Check sheet for the modelled part. Datum: model origin and axes. Units: mm. A direction names the side the tool comes from. Round coordinates to 2 decimals unless told otherwise and drop trailing zeros. Loops run counter-clockwise (first coordinate to the right, second up) from the corner with the lowest first, then second, coordinate; pieces in that order, holes last. Notation, with made-up numbers: (-29, 48) -> (-24, 48) arc R20 cw to (-24, 54) -> close; hole circle Ø6 at (77.5, 87.5). An arc over 180 degrees is marked (long way). Return JSON: item names as keys, results as strings.
from build123d import *

# Parameters (mm, degrees)
SKETCH_1_W                        = 13
SKETCH_1_H                        = 30
SM_BASE_FLANGE_1_DEPTH            = 1
SM_EDGE_FLANGE_1_STRIP_W          = 6
SM_EDGE_FLANGE_1_STRIP_H          = 1
SM_EDGE_FLANGE_1_STRIP_CUT_DEPTH  = 10
SM_EDGE_FLANGE_1_RELIEF_W         = 6.5
SM_EDGE_FLANGE_1_RELIEF_H         = 0.5
SM_EDGE_FLANGE_1_RELIEF_CUT_DEPTH = 1
SM_EDGE_FLANGE_1_DEPTH            = 10
SM_EDGE_FLANGE_1_PROFILE_R        = 1
SM_EDGE_FLANGE_1_PROFILE_R_2      = 0.75
SM_EDGE_FLANGE_1_FLAT_DEPTH       = 1
FILLET_1_R                        = 3
SKETCH_9_R                        = 1.6
CUT_EXTRUDE_1_DEPTH               = 18.615014781


# Sheet-metal steps are written as plain solids
with BuildPart() as part:
    # Sketch 1 → 基体-法兰1 (new body)
    with BuildSketch(Plane.XY):
        Rectangle(SKETCH_1_W, SKETCH_1_H)
    extrude(amount=-SM_BASE_FLANGE_1_DEPTH)

    # 边线-法兰1 strip (across the edge) → 边线-法兰1 strip cut (cut)
    with BuildSketch(Plane(origin=(-6.5, 5, -1), x_dir=(1, 0, 0), z_dir=(0, 1, 0))):
        with Locations((-1, -0.5)):
            Rectangle(SM_EDGE_FLANGE_1_STRIP_W, SM_EDGE_FLANGE_1_STRIP_H)
    sm_edge_flange_1_strip_cut = extrude(amount=SM_EDGE_FLANGE_1_STRIP_CUT_DEPTH, mode=Mode.SUBTRACT)

    # 边线-法兰1 relief (on the sheet) → 边线-法兰1 relief cut (cut)
    with BuildSketch(Plane(origin=(-4.5, 5, -1), x_dir=(1, 0, 0), z_dir=(0, 0, -1))):
        with Locations((-2.75, 0.25)):
            Rectangle(SM_EDGE_FLANGE_1_RELIEF_W, SM_EDGE_FLANGE_1_RELIEF_H)
    sm_edge_flange_1_relief_cut = extrude(amount=-SM_EDGE_FLANGE_1_RELIEF_CUT_DEPTH, mode=Mode.SUBTRACT)

    # 边线-法兰1 bend section (across the edge) → 边线-法兰1 (add)
    with BuildSketch(Plane(origin=(-6.5, 5, -1), x_dir=(1, 0, 0), z_dir=(0, 1, 0))):
        with BuildLine():
            Line((0, 1), (1, 1))
            ThreePointArc((1, 1), (1.292893219, 0.292893219), (2, 0))
            Line((2, 0), (2, -1))
            ThreePointArc((2, -1), (0.585786438, -0.414213562), (0, 1))
        make_face()
    sm_edge_flange_1 = extrude(amount=SM_EDGE_FLANGE_1_DEPTH)

    # 边线-法兰1 profile (on flange) → 边线-法兰1 flat (add)
    with BuildSketch(Plane(origin=(-6.5, 0, -1), x_dir=(0, -1, 0), z_dir=(1, 0, 0))):
        with BuildLine():
            Line((-15, 1), (-5, 1))
            Line((-5, 1), (-5, 3.360392195))
            ThreePointArc((-5, 3.360392195), (-5.453315717, 4.628370006), (-6.60776773, 5.321553546))
            Line((-6.60776773, 5.321553546), (-12.60776773, 6.521553546))
            ThreePointArc((-12.60776773, 6.521553546), (-14.267977811, 6.107076477), (-15, 4.560392195))
            Line((-15, 4.560392195), (-15, 1))
        make_face()
        with Locations((-13, 2.5)):
            Circle(SM_EDGE_FLANGE_1_PROFILE_R, mode=Mode.SUBTRACT)
        with Locations((-7, 3.360392195)):
            Circle(SM_EDGE_FLANGE_1_PROFILE_R_2, mode=Mode.SUBTRACT)
    sm_edge_flange_1_flat = extrude(amount=SM_EDGE_FLANGE_1_FLAT_DEPTH)

    # 镜向1: 边线-法兰1 strip cut, 边线-法兰1 relief cut, 边线-法兰1, 边线-法兰1 flat across plane
    add(sm_edge_flange_1_strip_cut.mirror(Plane(origin=(0, 0, 0), x_dir=(0, 0, 1), z_dir=(1, 0, 0))), mode=Mode.SUBTRACT)
    add(sm_edge_flange_1_relief_cut.mirror(Plane(origin=(0, 0, 0), x_dir=(0, 0, 1), z_dir=(1, 0, 0))), mode=Mode.SUBTRACT)
    add(sm_edge_flange_1.mirror(Plane(origin=(0, 0, 0), x_dir=(0, 0, 1), z_dir=(1, 0, 0))))
    add(sm_edge_flange_1_flat.mirror(Plane(origin=(0, 0, 0), x_dir=(0, 0, 1), z_dir=(1, 0, 0))))

    # 圆角1
    fillet_1_edges = [part.edges().sort_by_distance(p)[0] for p in [
        (6.5, -15, -0.5),
        (-6.5, -15, -0.5),
    ]]
    fillet(fillet_1_edges, radius=FILLET_1_R)

    # 草图9 → 切除-拉伸1 (cut, through all)
    with BuildSketch(Plane(origin=(0, 0, -1), x_dir=(-1, 0, 0), z_dir=(0, 0, -1))):
        with Locations((0, 8)):
            Circle(SKETCH_9_R)
        with Locations((0, -5)):
            Circle(SKETCH_9_R)
    extrude(amount=-CUT_EXTRUDE_1_DEPTH, mode=Mode.SUBTRACT)


solid = part.part
Q1. Section check C-C (y = -5). Record the boundary of the cut face in (x, z).
Results list:
{"outline": "(-6.5, -1) -> (-1.6, -1) -> (-1.6, 0) -> (-6.5, 0) -> close; (1.6, -1) -> (6.5, -1) -> (6.5, 0) -> (1.6, 0) -> close"}
Q2. Section check A-A (x = 0). Record the boundary of the cut face in (y, z), then the cut area to 3 significant figures.
Results list:
{"outline": "(-15, -1) -> (-6.6, -1) -> (-6.6, 0) -> (-15, 0) -> close; (-3.4, -1) -> (6.4, -1) -> (6.4, 0) -> (-3.4, 0) -> close; (9.6, -1) -> (15, -1) -> (15, 0) -> (9.6, 0) -> close", "area": "23.6 mm^2"}
Q3. Draft check along X on faces 1 (the flat face through (-5.5, 10, -5)), 2 (the cylindrical face through (-5.9, 9.93, -0.57)), 3 (the flat face through (0, -15, -0.5)). Enter one of: released by +X, released by -X, zero draft, split by the parting line, or undercut.
Results list:
{"face 1": "undercut", "face 2": "released by -X", "face 3": "zero draft"}
Q4. Tool access check on faces 4 (the flat face through (-5.3, 4.5, -0.5)), 5 (the cylindrical face through (5.64, -14.1, -0.51)), 6 (the flat face through (5.5, 10, -5)). Record the directions out of +Z, -Z, +X, -X, +Y, -Y that give a thin tool (end or side, any length) a straight path to the whole face; none if there is none.
Results list:
{"face 4": "+Z, -Z, -X", "face 5": "+Z, -Z, +X, -Y", "face 6": "-Z, +Y, -Y"}
Q5. Section check D-D (y = 10). Record the boundary of the cut face in (x, z).
Results list:
{"outline": "(-6.5, -7) -> (-5.5, -7) -> (-5.5, -2) arc R1 cw to (-4.5, -1) -> (4.5, -1) arc R1 cw to (5.5, -2) -> (5.5, -7) -> (6.5, -7) -> (6.5, -2) arc R2 ccw to (4.5, 0) -> (-4.5, 0) arc R2 ccw to (-6.5, -2) -> close"}
Q6. Material ranges on line 1 (Y direction, x = 0, z = -0.45); line 2 (X direction, y = 8.5, z = -5.5); line 3 (Y direction, x = -5.95, z = -3.5), recorded low to high.
Results list:
{"line 1": "-15 to -6.6, -3.4 to 6.4, 9.6 to 15", "line 2": "-6.5 to -5.5, 5.5 to 6.5", "line 3": "5 to 12, 14 to 15"}
Q7. Section check B-B (y = 13). Record the boundary of the cut face in (x, z), then the cut area to 3 significant figures.
Results list:
{"outline": "(-6.5, -7.56) -> (-5.5, -7.56) -> (-5.5, -4.5) -> (-6.5, -4.5) -> close; (-6.5, -2.5) -> (-5.5, -2.5) -> (-5.5, -2) arc R1 cw to (-4.5, -1) -> (4.5, -1) arc R1 cw to (5.5, -2) -> (5.5, -2.5) -> (6.5, -2.5) -> (6.5, -2) arc R2 ccw to (4.5, 0) -> (-4.5, 0) arc R2 ccw to (-6.5, -2) -> close; (5.5, -7.56) -> (6.5, -7.56) -> (6.5, -4.5) -> (5.5, -4.5) -> close", "area": "20.8 mm^2"}
Q8. Go/stop test with flat-tipped pins: pin 1 (3 mm diameter, centred on x = 5, z = -3, fed in from -Y); pin 2 (3 mm diameter, centred on x = -5.5, z = -2, fed in from -Y). Record where each tip stops, or that it passes through.
Results list:
{"pin 1": "y = 5", "pin 2": "y = -14.87"}
